```python
from build123d import *

# Parameters (mm, degrees)
SKETCH1_W           = 7.1
SKETCH1_H           = 3
BOSS_EXTRUDE1_DEPTH = 20
SKETCH2_R           = 1.55
CUT_EXTRUDE1_DEPTH  = 20
FILLET1_R           = 5
CHAMFER1_SIZE       = 3
CHAMFER2_SIZE       = 1.662927154
CHAMFER2_SIZE_2     = 3


# Some blends are built 0.0001 mm under size
with BuildPart() as part:
    # Sketch1 → Boss-Extrude1 (new body)
    with BuildSketch(Plane(origin=(0, 0, 0), x_dir=(0, 0, -1), z_dir=(1, 0, 0))):
        with Locations((3.55, -1.5)):
            Rectangle(SKETCH1_W, SKETCH1_H)
        Polygon((22.1, -3), (7.1, -3), (5.1, -3), (5.1, -5.1), (22.1, -5.1), align=None)
    extrude(amount=BOSS_EXTRUDE1_DEPTH)

    # Sketch2 → Cut-Extrude1 (cut)
    with BuildSketch(Plane(origin=(0, -3, 0), x_dir=(1, 0, 0), z_dir=(0, 1, 0))):
        with Locations(Location((10, 17.1, 0), (0, 0, 270))):
            Circle(SKETCH2_R)
    extrude(amount=-CUT_EXTRUDE1_DEPTH, mode=Mode.SUBTRACT)

    # Fillet1
    fillet1_edges = [part.edges().sort_by_distance(p)[0] for p in [
        (0, -4.05, -22.1),
        (20, -4.05, -22.1),
    ]]
    fillet(fillet1_edges, radius=FILLET1_R)

    # Chamfer1
    chamfer1_edges = [part.edges().sort_by_distance(p)[0] for p in [
        (10, -3, -7.1),
    ]]
    chamfer(chamfer1_edges, length=CHAMFER1_SIZE - 0.0001)  # a hair under: the kernel refuses the full size

    # Chamfer2
    # the kernel refuses this chamfer: 3, 1.662927154 mm, written as the material it takes off along each edge
    with BuildSketch(Plane(origin=(-7.763748365, 0, 0), x_dir=(0, 0.06086775916528878, -0.9981458389905739), z_dir=(1, 0, 0))) as chamfer2_piece_1:
        Polygon((CHAMFER2_SIZE * 0.998145839206, -CHAMFER2_SIZE * 0.0608677591784), (-CHAMFER2_SIZE_2 * 0.0608677591653, -CHAMFER2_SIZE_2 * 0.998145838991), (0, 0), align=None)
    extrude(amount=35.527496731, mode=Mode.SUBTRACT)


solid = part.part
```
Work out the finished part from the listing and answer in its coordinate system (mm). A direction names the side the tool comes from. Round coordinates to 2 decimals unless told otherwise and drop trailing zeros. Write each loop counter-clockwise with the first axis right and the second up, starting at its lowest first coordinate (ties: lowest second). Pieces come first, ordered by that corner, then holes. Notation, with made-up numbers: (6.5, 83) - (47.5, 83) arc R12 ccw to (47.5, 93) - close; hole circle Ø2 at (24.5, 79). An arc over 180 degrees is marked (long way). Return JSON: item names as keys, results as strings. Group by question number.
Q1. The mould has two halves that part along X. Classify faces 1 (the flat face through (20, -3, -8)), 2 (the flat face through (10, -3, -15)), 3 (the cylindrical face through (10.466, -4.035, -15.622)): released by +X, released by -X, zero draft, split by the parting line, or undercut.
Q2. Find the intervals of material crossed by L1, parallel to X at y = -4.25, z = -17.1; L2, parallel to Y at x = 11, z = -20; L3, parallel to Z at x = 10.25, y = -3.75, in increasing order.
Q3. For faces 4 (the flat face through (10, -4, -22.1)), 5 (the flat face through (10, -3, -3)), determine the directions among +Z, -Z, +X, -X, +Y, -Y from which every point of the face is accessible in a straight line to the end or side of a thin tool.
Q4. The part is cut by section B-B on y = -4.75. Write down the section's boundary in (x, z).
Q5. The part is cut by section C-C on z = -17.5. Write down the section's boundary in (x, y).
Q6. Each of these flat-tipped pins is pushed along its axis until it touches: pin 1 Ø2 at (x, y) = (13.5, -0.5) entering from +Z; pin 2 Ø4 at (x, z) = (14.5, -2.5) entering from -Y; pin 3 Ø4 at (x, z) = (10, -17.1) entering from +Y; pin 4 Ø3 at (y, z) = (-2.5, -17.5) entering from +X. Where does it stop, or does it pass through?
Solved:
{
 "1": {"face 1": "released by +X", "face 2": "zero draft", "face 3": "undercut"},
 "2": {"L1": "0 to 8.45, 11.55 to 20", "L2": "-5.1 to -3", "L3": "-22.1 to -18.63, -15.57 to -5.1"},
 "3": {"face 4": "-Z, +X, -X, +Y, -Y", "face 5": "+Z, +X, -X, -Y"},
 "4": {"outline": "(0, -17.1) arc R5 ccw to (5, -22.1) - (15, -22.1) arc R5 ccw to (20, -17.1) - (20, -5.1) - (0, -5.1) - close; hole circle Ø3.1 at (10, -17.1)"},
 "5": {"outline": "(0.02, -5.1) - (8.5, -5.1) - (8.5, -3) - (0.02, -3) - close; (11.5, -5.1) - (19.98, -5.1) - (19.98, -3) - (11.5, -3) - close"},
 "6": {"pin 1": "z = -0.83", "pin 2": "y = -3", "pin 3": "y = -3", "pin 4": "x = 20"}
}
